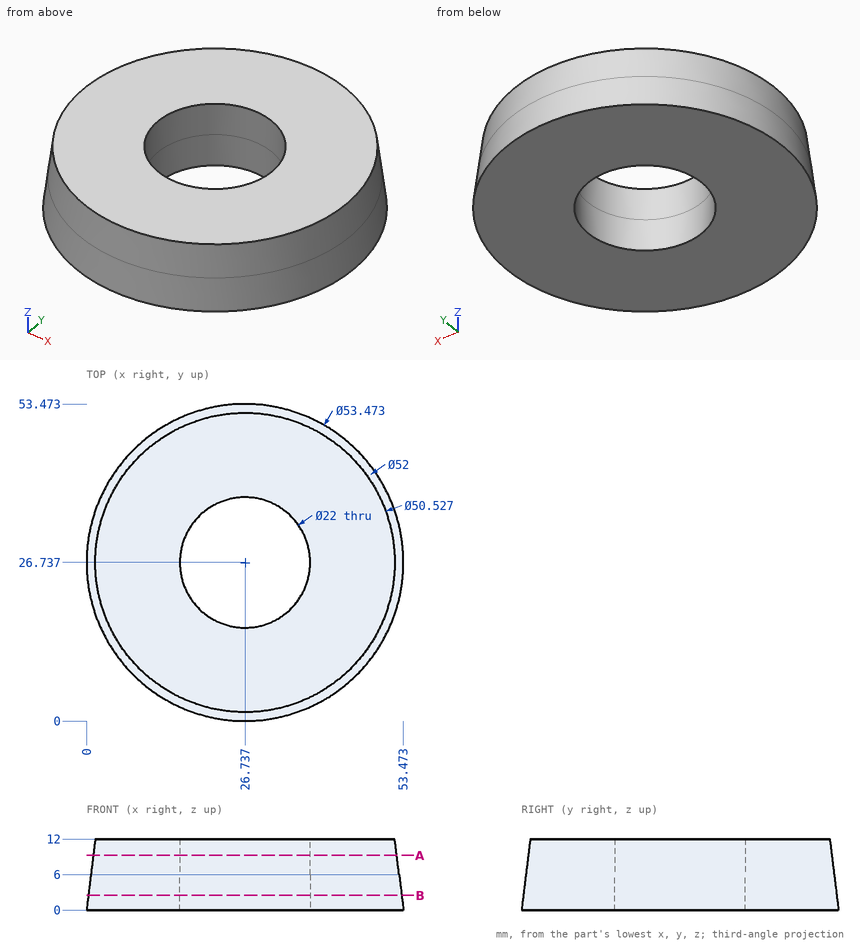
Source: three-view drawing plus pictorial views. Frame: mm from the lowest corner of the part. Round coordinates to 2 decimals unless told otherwise and drop trailing zeros. Order: outer loops, then holes, each group sorted by start corner. A loop starts at its lowest first (then second) coordinate and runs counter-clockwise, first axis right, second up. Notation, with made-up numbers: (-28, 44.25) - (7, 44.25) arc R20 cw to (7, 62.25) - close; hole circle Ø3 at (33, -33.5). An arc over 180 degrees is marked (long way). Use a Markdown table: item, result.
1. Section A-A on z = 9.25. Return the cut outline in (x, y), then the cut area to 3 significant figures.
Evaluation:
| item | result |
|---|---|
| outline | circle Ø51.2 at (26.74, 26.74); hole circle Ø22 at (26.74, 26.74) |
| area | 1,680 mm^2 |
2. Section B-B on z = 2.5. Return the cut outline in (x, y), then the cut area to 3 significant figures.
Evaluation:
| item | result |
|---|---|
| outline | circle Ø52.86 at (26.74, 26.74); hole circle Ø22 at (26.74, 26.74) |
| area | 1,810 mm^2 |
3. First-contact query: pin 1 (1 mm diameter, centred on x = 44.5, z = 10, fed in from +Y) (1 decimal); pin 2 (1.5 mm diameter, centred on x = 11.5, z = 3.5, fed in from +Y); pin 3 (1.5 mm diameter, centred on x = 33.5, z = 4, fed in from +Y). Flat tips, straight axial feed; report the tip coordinate or a pass-through.
Evaluation:
| item | result |
|---|---|
| pin 1 | y = 45.5 |
| pin 2 | y = 48.71 |
| pin 3 | y = 52.31 |
4. Material intervals for probe 1 along Y at (x, z) = (24.5, 7); probe 2 along Y at (x, z) = (18.5, 10.25) (1 decimal); probe 3 along X at (y, z) = (33, 7.5) (1 decimal), sorted ascending.
Evaluation:
| item | result |
|---|---|
| probe 1 | 0.96 to 15.97, 37.51 to 52.52 |
| probe 2 | 2.6 to 19.4, 34 to 50.8 |
| probe 3 | 1.7 to 17.7, 35.8 to 51.8 |
